from build123d import *

# Parameters (mm, degrees)
SKETCH006_W                = 19.6
SKETCH006_H                = 17
PAD001_DEPTH               = 0.5
SKETCH011_W                = 0.5
SKETCH011_H                = 17
PAD002_DEPTH               = 1.5
SKETCH012_W                = 0.5
SKETCH012_H                = 2
PAD003_DEPTH               = 5.2
SKETCH012_MIRRORED008_2_W  = 0.5
SKETCH012_MIRRORED008_2_H  = 2
PAD003_MIRRORED008_2_DEPTH = 5.2
PAD004_DEPTH               = 0.5
PAD004_MIRRORED010_2_DEPTH = 0.5
FILLET_R                   = 0.5


with BuildPart() as part:
    # Sketch006 → Pad001 (new body)
    with BuildSketch(Plane.XY.offset(15.2)):
        Rectangle(SKETCH006_W, SKETCH006_H)
    extrude(amount=PAD001_DEPTH)

    # Sketch011 (on Face5 of Pad001) → Pad002 (join)
    with BuildSketch(Plane(origin=(0, 0, 15.2), x_dir=(1, 0, 0), z_dir=(0, 0, -1))):
        with Locations((-9.55, 0)):
            Rectangle(SKETCH011_W, SKETCH011_H)
    pad002 = extrude(amount=PAD002_DEPTH)

    # Mirrored007: Pad002 across YZ
    add(pad002.mirror(Plane.YZ))

    # Sketch012 (on Face5 of Mirrored007) → Pad003 (join)
    with BuildSketch(Plane(origin=(0, 0, 13.7), x_dir=(1, 0, 0), z_dir=(0, 0, -1))):
        with Locations((-9.55, 5.5)):
            Rectangle(SKETCH012_W, SKETCH012_H)
    pad003 = extrude(amount=PAD003_DEPTH)

    # Sketch012 Mirrored008 2 → Pad003 Mirrored008 2 (add)
    with BuildSketch(Plane(origin=(0, 0, 13.7), x_dir=(-1, 0, 0), z_dir=(0, 0, 1))):
        with Locations((-9.55, 5.5)):
            Rectangle(SKETCH012_MIRRORED008_2_W, SKETCH012_MIRRORED008_2_H)
    pad003_mirrored008_2 = extrude(amount=-PAD003_MIRRORED008_2_DEPTH)

    # Mirrored009: Pad003, Pad003 Mirrored008 2 across XZ
    add(pad003.mirror(Plane.XZ))
    add(pad003_mirrored008_2.mirror(Plane.XZ))

    # Sketch013 (on Face24 of MultiTransform001) → Pad004 (join)
    with BuildSketch(Plane(origin=(-9.8, 0, 0), x_dir=(0, -1, 0), z_dir=(-1, 0, 0))):
        with BuildLine():
            ThreePointArc((-7.247226, 7.814702), (-7.306335, 7.663488), (-7.182824, 7.558111))
            add(Edge.make_bspline(
                [(-7.182824, 7.558111), (-5.976509, 7.451929), (-5.547279, 8.5)],
                knots=[1.033239, 1.033239, 1.033239, 2.478771, 2.478771, 2.478771], degree=2, weights=[1, 0.749979, 1]))
            Line((-5.547279, 8.5), (-6.5, 8.5))
            add(Edge.make_bspline(
                [(-7.247226, 7.814702), (-6.810749, 8.100432), (-6.5, 8.5)],
                knots=[1.339981, 1.339981, 1.339981, 1.941601, 1.941601, 1.941601], degree=2, weights=[1, 0.955097, 1]))
        make_face()
        with BuildLine():
            add(Edge.make_bspline(
                [(-5.452721, 8.5), (-5.023491, 7.451929), (-3.817176, 7.558111)],
                knots=[3.804414, 3.804414, 3.804414, 5.249946, 5.249946, 5.249946], degree=2, weights=[1, 0.749979, 1]))
            ThreePointArc((-3.817176, 7.558111), (-3.693665, 7.663488), (-3.752774, 7.814702))
            add(Edge.make_bspline(
                [(-4.5, 8.5), (-4.189251, 8.100432), (-3.752774, 7.814702)],
                knots=[4.341585, 4.341585, 4.341585, 4.943204, 4.943204, 4.943204], degree=2, weights=[1, 0.955097, 1]))
            Line((-4.5, 8.5), (-5.452721, 8.5))
        make_face()
    pad004 = extrude(amount=-PAD004_DEPTH)

    # Sketch013 Mirrored010 2 → Pad004 Mirrored010 2 (add)
    with BuildSketch(Plane(origin=(9.8, 0, 0), x_dir=(0, -1, 0), z_dir=(-1, 0, 0))):
        with BuildLine():
            ThreePointArc((-7.247226, 7.814702), (-7.306335, 7.663488), (-7.182824, 7.558111))
            add(Edge.make_bspline(
                [(-7.182824, 7.558111), (-5.976509, 7.451929), (-5.547279, 8.5)],
                knots=[1.033239, 1.033239, 1.033239, 2.478771, 2.478771, 2.478771], degree=2, weights=[1, 0.749979, 1]))
            Line((-5.547279, 8.5), (-6.5, 8.5))
            add(Edge.make_bspline(
                [(-7.247226, 7.814702), (-6.810749, 8.100432), (-6.5, 8.5)],
                knots=[1.339981, 1.339981, 1.339981, 1.941601, 1.941601, 1.941601], degree=2, weights=[1, 0.955097, 1]))
        make_face()
        with BuildLine():
            add(Edge.make_bspline(
                [(-5.452721, 8.5), (-5.023491, 7.451929), (-3.817176, 7.558111)],
                knots=[3.804414, 3.804414, 3.804414, 5.249946, 5.249946, 5.249946], degree=2, weights=[1, 0.749979, 1]))
            ThreePointArc((-3.817176, 7.558111), (-3.693665, 7.663488), (-3.752774, 7.814702))
            add(Edge.make_bspline(
                [(-4.5, 8.5), (-4.189251, 8.100432), (-3.752774, 7.814702)],
                knots=[4.341585, 4.341585, 4.341585, 4.943204, 4.943204, 4.943204], degree=2, weights=[1, 0.955097, 1]))
            Line((-4.5, 8.5), (-5.452721, 8.5))
        make_face()
    pad004_mirrored010_2 = extrude(amount=PAD004_MIRRORED010_2_DEPTH)

    # Mirrored011: Pad004, Pad004 Mirrored010 2 across XZ
    add(pad004.mirror(Plane.XZ))
    add(pad004_mirrored010_2.mirror(Plane.XZ))

    # Fillet
    fillet_edges = [part.edges().sort_by_distance(p)[0] for p in [
        (-9.8, 0, 15.7),
        (9.8, 0, 15.7),
    ]]
    fillet(fillet_edges, radius=FILLET_R)


solid = part.part
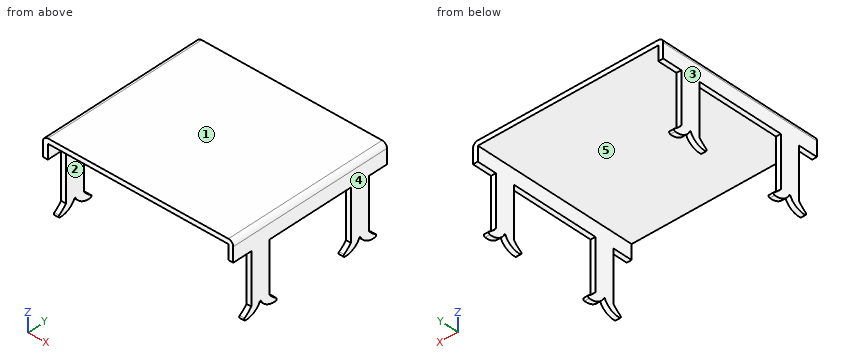
Read the model definition and answer for the solid it produces. Units are mm, in the model's axes. Face numbers are marked on the shaded views. A direction names the side the tool comes from. Round coordinates to 2 decimals unless told otherwise and drop trailing zeros. Order: outer loops, then holes, each group sorted by start corner. A loop starts at its lowest first (then second) coordinate and runs counter-clockwise, first axis right, second up.
1) Straight lines are drawn through the part: L1, parallel to X at y = -7.5, z = 14.75; L2, parallel to Z at x = -8.5, y = -7; L3, parallel to X at y = -0.5, z = 15.5. For each, find the intervals that lie inside material, in ascending order.
2) The part is cut by section C-C on x = 1.75. Write down the section's boundary in (y, z), plus the area to 3 significant figures.
3) The mould has two halves that part along X. Classify the marked faces 1, 2 and 3: released by +X, released by -X, zero draft, split by the parting line, or undercut.
4) Flat-ended cylindrical pins translate along their axes: pin 1 (3 mm diameter, centred on x = -0.5, y = 0, fed in from -Z); pin 2 (4 mm diameter, centred on x = 1, z = 12.5, fed in from +Y); pin 3 (0.6 mm diameter, centred on x = -9.5, y = -8, fed in from -Z). Find the tip coordinate at first contact, or state that the pin passes through.
5) For the marked faces 4 and 5, determine the directions among +Z, -Z, +X, -X, +Y, -Y from which every point of the face is accessible in a straight line to the end or side of a thin tool.
6) The part is cut by section A-A on z = 12.25. Write down the section's boundary in (x, y), plus the area to 3 significant figures.
7) The part is cut by section D-D on y = 4.25. Give the number of separate pieces and of enclosed holes in the cut face, plus the area to 3 significant figures.
8) The part is cut by section B-B on y = 1.75. Write down the section's boundary in (x, z), plus the area to 3 significant figures.
Resolved:
1. L1: x = -9.8 to -9.3, 9.3 to 9.8
1. L2: z = 15.2 to 15.7
1. L3: x = -9.7 to 9.7
2. outline: (-8.5, 15.2) - (8.5, 15.2) - (8.5, 15.7) - (-8.5, 15.7) - close
2. area: 8.50 mm2
3. face 1: zero draft
3. face 2: undercut
3. face 3: released by -X
4. pin 1: stops at z = 15.2
4. pin 2: passes through
4. pin 3: stops at z = 13.7
5. face 4: +Z, -Z, +X, +Y, -Y
5. face 5: -Z, +Y, -Y
6. outline: (-9.8, -6.5) - (-9.3, -6.5) - (-9.3, -4.5) - (-9.8, -4.5) - close; (-9.8, 4.5) - (-9.3, 4.5) - (-9.3, 6.5) - (-9.8, 6.5) - close; (9.3, -6.5) - (9.8, -6.5) - (9.8, -4.5) - (9.3, -4.5) - close; (9.3, 4.5) - (9.8, 4.5) - (9.8, 6.5) - (9.3, 6.5) - close
6. area: 4.00 mm2
7. separate pieces: 3
7. enclosed holes: 0
7. area: 11.8 mm2
8. outline: (-9.8, 13.7) - (-9.3, 13.7) - (-9.3, 15.2) - (9.3, 15.2) - (9.3, 13.7) - (9.8, 13.7) - (9.8, 15.2) arc R0.5 ccw to (9.3, 15.7) - (-9.3, 15.7) arc R0.5 ccw to (-9.8, 15.2) - close
8. area: 11.2 mm2
